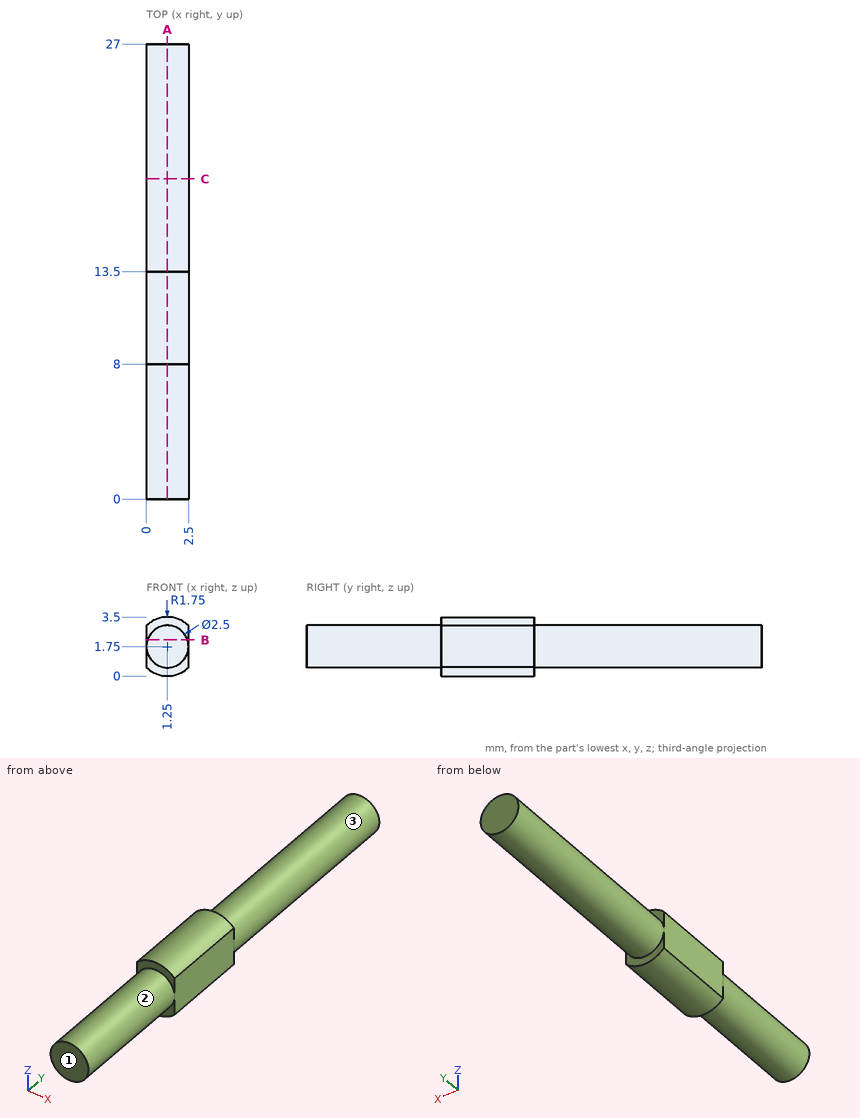
Design review of the part shown in the three views and the two pictorial views. Dimensions are in mm from the part's minimum x, y and z. A direction names the side the tool comes from. Round coordinates to 2 decimals unless told otherwise and drop trailing zeros. Order: outer loops, then holes, each group sorted by start corner. A loop starts at its lowest first (then second) coordinate and runs counter-clockwise, first axis right, second up.
Q1. Wall thickness on line 1 (Y direction, x = 1.2, z = 3.25); line 2 (X direction, y = 7.25, z = 1.8); line 3 (Z direction, x = 2.1, y = 7.25): over which ranges is each line inside the solid? List them lowest first.
Findings below:
line 1: y = 8 to 13.5
line 2: x = 0 to 2.5
line 3: z = 0.83 to 2.67
Q2. We need section C-C, the plane y = 19. Give the boundary of the cut face in (x, z).
Findings below:
outline: circle Ø2.5 at (1.25, 1.75)
Q3. Insertion check: P1, Ø1, axis at x = 2, y = 17, coming from the +Z side. The pin has a flat end and moves straight along its axis. Give the tip position at first contact, or say it passes through.
Findings below:
P1: stops at z = 2.97
Q4. Machinability: for the marked faces 1, 2 and 3, which of the approach directions +Z, -Z, +X, -X, +Y, -Y give a long, thin tool a straight path to every point of the face, cutting with its end or side? Answer none if there is none.
Findings below:
face 1: +Z, -Z, +X, -X, -Y
face 2: -Y
face 3: +Y
Q5. We need section B-B, the plane z = 2.15. Give the boundary of the cut face in (x, y), plus the area to 3 significant figures.
Findings below:
outline: (0, 8) - (0.07, 8) - (0.07, 0) - (2.43, 0) - (2.43, 8) - (2.5, 8) - (2.5, 13.5) - (2.43, 13.5) - (2.43, 27) - (0.07, 27) - (0.07, 13.5) - (0, 13.5) - close
area: 64.7 mm2
Q6. We need section A-A, the plane x = 1.25. Give the boundary of the cut face in (y, z), plus the area to 3 significant figures.
Findings below:
outline: (0, 0.5) - (8, 0.5) - (8, 0) - (13.5, 0) - (13.5, 0.5) - (27, 0.5) - (27, 3) - (13.5, 3) - (13.5, 3.5) - (8, 3.5) - (8, 3) - (0, 3) - close
area: 73.0 mm2
